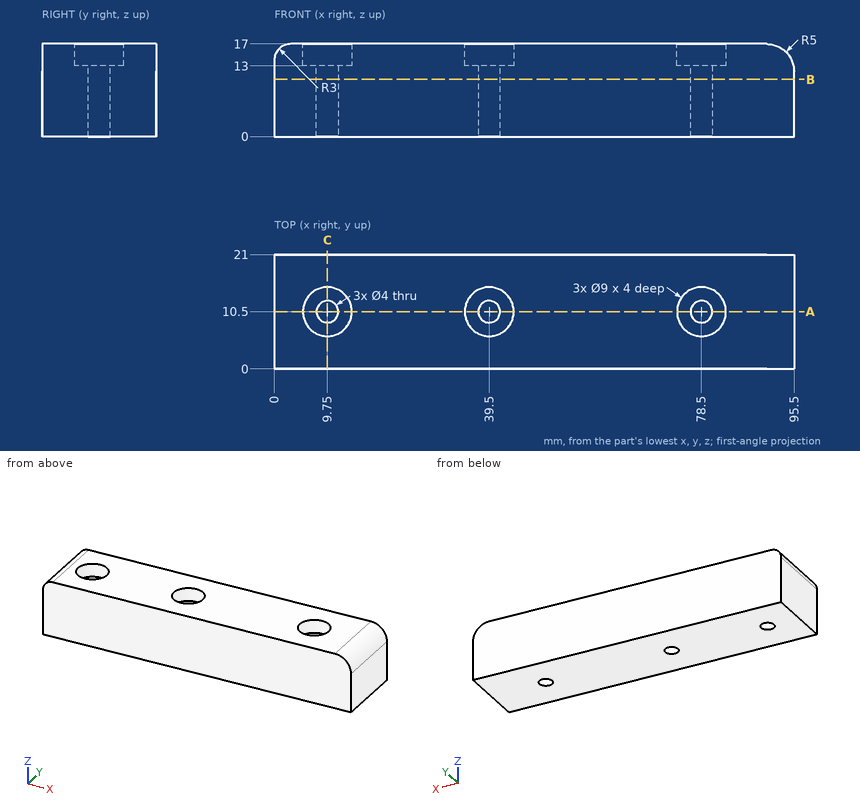
Input: dimensioned drawing with shaded views. Units: mm. Origin: part minimum x, y, z. Give positions to 0.01 mm unless a question says otherwise; leave off trailing zeros. Write each loop counter-clockwise with the first axis right and the second up, starting at its lowest first coordinate (ties: lowest second). Pieces come first, ordered by that corner, then holes.
1. Line query: probe 1 along X at (y, z) = (9, 8.75); probe 2 along X at (y, z) = (8.75, 5.5); probe 3 along Y at (x, z) = (9.75, 4.25). Output: solid intervals per line, ascending.
2. Section query B-B, the plane z = 10.5. Return loops of the section in (x, y), then the cut area to 3 significant figures.
3. Pin query (flat end, axial travel): P1, Ø3.5, axis at x = 9.75, y = 10.5, coming from the -Z side; P2, Ø7, axis at x = 79, y = 10.5, coming from the +Z side. Return the tip coordinate at first contact, or that it passes through.
4. Section query C-C, the plane x = 9.75. Return loops of the section in (y, z), then the cut area to 3 significant figures.
5. Section query A-A, the plane y = 10.5. Count the separate pieces of the cut face and the enclosed holes in it, then the cut area to 3 significant figures.
Computed:
1. probe 1: x = 0 to 8.43, 11.07 to 38.18, 40.82 to 77.18, 79.82 to 95.5
1. probe 2: x = 0 to 8.78, 10.72 to 38.53, 40.47 to 77.53, 79.47 to 95.5
1. probe 3: y = 0 to 8.5, 12.5 to 21
2. outline: (0, 0) - (95.5, 0) - (95.5, 21) - (0, 21) - close; hole circle Ø4 at (9.75, 10.5); hole circle Ø4 at (39.5, 10.5); hole circle Ø4 at (78.5, 10.5)
2. area: 1,970 mm2
3. P1: passes through
3. P2: stops at z = 13
4. outline: (0, 0) - (8.5, 0) - (8.5, 13) - (6, 13) - (6, 17) - (0, 17) - close; (12.5, 0) - (21, 0) - (21, 17) - (15, 17) - (15, 13) - (12.5, 13) - close
4. area: 269 mm2
5. separate pieces: 4
5. enclosed holes: 0
5. area: 1,350 mm2
